CAD build for the part. Positions are in the model's coordinates, mm. A direction names the side the tool comes from. Coordinates: 2 decimals unless noted, no trailing zeros. Write each loop counter-clockwise with the first axis right and the second up, starting at its lowest first coordinate (ties: lowest second). Pieces come first, ordered by that corner, then holes. Notation, with made-up numbers: M -7,-18.5 L 8,-18.5 A16 cw 8,6.5 Z; hole C 3.5,16 d7. An arc over 180 degrees is marked long. Answer as CSV lines item,"result". Start each with the question number.
```python
from build123d import *

# Parameters (mm, degrees)
SKETCH1_R           = 3.5
SKETCH1_R_2         = 1.5
SKETCH1_R_3         = 1.1
EXTRUDE_1_DEPTH     = 3
CUT_EXTRUDE_1_DEPTH = 1.5


with BuildPart() as part:
    # Sketch1 → Бобышка-Вытянуть1 (new body)
    with BuildSketch(Plane.XY):
        with BuildLine():
            Line((-24.498196466, 18.686253871), (-28.812938034, 21.763271713))
            ThreePointArc((-28.812938034, 21.763271713), (-34.033313652, 22.967935089), (-38.576502294, 20.128397731))
            Line((-38.576502294, 20.128397731), (-42.0602267, 15.24335277))
            ThreePointArc((-42.0602267, 15.24335277), (-43.264890076, 10.022977152), (-40.425352718, 5.47978851))
            Line((-40.425352718, 5.47978851), (-36.440527218, 2.638047245))
            ThreePointArc((-36.440527218, 2.638047245), (-34.281914219, 0.144259766), (-33.504872357, -3.061171876))
            Line((-33.504872357, -3.061171876), (-33.504872357, -48.061171876))
            ThreePointArc((-33.504872357, -48.061171876), (-34.969338451, -51.596705782), (-38.504872357, -53.061171876))
            Line((-38.504872357, -53.061171876), (-42.504872357, -53.061171876))
            ThreePointArc((-42.504872357, -53.061171876), (-47.454619825, -55.111424407), (-49.504872357, -60.061171876))
            Line((-49.504872357, -60.061171876), (-49.500334917, -60.235639257))
            Line((-49.500334917, -60.235639257), (-49.500334917, -66.108369799))
            Line((-49.500334917, -66.108369799), (-49.504872357, -66.28283718))
            ThreePointArc((-49.504872357, -66.28283718), (-47.454619825, -71.232584649), (-42.504872357, -73.28283718))
            Line((-42.504872357, -73.28283718), (-38.504872357, -73.28283718))
            ThreePointArc((-38.504872357, -73.28283718), (-34.969338451, -74.747303275), (-33.504872357, -78.28283718))
            Line((-33.504872357, -78.28283718), (-33.504872357, -123.28283718))
            ThreePointArc((-33.504872357, -123.28283718), (-34.281914219, -126.488268823), (-36.440527218, -128.982056301))
            Line((-36.440527218, -128.982056301), (-40.425352718, -131.823797566))
            ThreePointArc((-40.425352718, -131.823797566), (-43.264890076, -136.366986209), (-42.0602267, -141.587361827))
            Line((-42.0602267, -141.587361827), (-38.576502294, -146.472406787))
            ThreePointArc((-38.576502294, -146.472406787), (-34.033313652, -149.311944145), (-28.812938034, -148.107280769))
            Line((-28.812938034, -148.107280769), (-24.498196466, -145.030262927))
            ThreePointArc((-24.498196466, -145.030262927), (-21.740151192, -143.647892601), (-18.691989124, -143.172004528))
            Line((-18.691989124, -143.172004528), (46.687073776, -143.172004528))
            ThreePointArc((46.687073776, -143.172004528), (49.735235844, -143.647892601), (52.493281118, -145.030262927))
            Line((52.493281118, -145.030262927), (56.808022686, -148.107280769))
            ThreePointArc((56.808022686, -148.107280769), (62.028398304, -149.311944145), (66.571586947, -146.472406787))
            Line((66.571586947, -146.472406787), (70.055311352, -141.587361827))
            ThreePointArc((70.055311352, -141.587361827), (71.259974728, -136.366986209), (68.42043737, -131.823797566))
            Line((68.42043737, -131.823797566), (64.43561187, -128.982056301))
            ThreePointArc((64.43561187, -128.982056301), (62.276998871, -126.488268823), (61.499957009, -123.28283718))
            Line((61.499957009, -123.28283718), (61.499957009, -78.28283718))
            ThreePointArc((61.499957009, -78.28283718), (62.964423103, -74.747303275), (66.499957009, -73.28283718))
            Line((66.499957009, -73.28283718), (70.499957009, -73.28283718))
            ThreePointArc((70.499957009, -73.28283718), (75.449704478, -71.232584649), (77.499957009, -66.28283718))
            Line((77.499957009, -66.28283718), (77.495419569, -66.108369799))
            Line((77.495419569, -66.108369799), (77.495419569, -60.235639257))
            Line((77.495419569, -60.235639257), (77.499957009, -60.061171876))
            ThreePointArc((77.499957009, -60.061171876), (75.449704478, -55.111424407), (70.499957009, -53.061171876))
            Line((70.499957009, -53.061171876), (66.499957009, -53.061171876))
            ThreePointArc((66.499957009, -53.061171876), (62.964423103, -51.596705782), (61.499957009, -48.061171876))
            Line((61.499957009, -48.061171876), (61.499957009, -3.061171876))
            ThreePointArc((61.499957009, -3.061171876), (62.276998871, 0.144259766), (64.43561187, 2.638047245))
            Line((64.43561187, 2.638047245), (68.42043737, 5.47978851))
            ThreePointArc((68.42043737, 5.47978851), (71.259974728, 10.022977152), (70.055311352, 15.24335277))
            Line((70.055311352, 15.24335277), (66.571586947, 20.128397731))
            ThreePointArc((66.571586947, 20.128397731), (62.028398304, 22.967935089), (56.808022686, 21.763271713))
            Line((56.808022686, 21.763271713), (52.493281118, 18.686253871))
            ThreePointArc((52.493281118, 18.686253871), (49.735235844, 17.303883544), (46.687073776, 16.827995472))
            Line((46.687073776, 16.827995472), (1.690542794, 16.827995472))
            ThreePointArc((1.690542794, 16.827995472), (1.120947956, 16.649921089), (0.754213617, 16.179118913))
            Line((0.754213617, 16.179118913), (-0.502457674, 12.827995472))
            Line((-0.502457674, 12.827995472), (0.997542326, 12.827995472))
            Line((0.997542326, 12.827995472), (0.997542326, 7.827995472))
            ThreePointArc((0.997542326, 7.827995472), (0.704649107, 7.120888691), (-0.002457674, 6.827995472))
            Line((-0.002457674, 6.827995472), (-1.002457674, 6.827995472))
            ThreePointArc((-1.002457674, 6.827995472), (-1.709564455, 7.120888691), (-2.002457674, 7.827995472))
            Line((-2.002457674, 7.827995472), (-2.002457674, 15.827995472))
            ThreePointArc((-2.002457674, 15.827995472), (-2.295350893, 16.535102253), (-3.002457674, 16.827995472))
            Line((-3.002457674, 16.827995472), (-18.691989124, 16.827995472))
            ThreePointArc((-18.691989124, 16.827995472), (-21.740151192, 17.303883544), (-24.498196466, 18.686253871))
        make_face()
        with Locations((68.745419569, -63.172004528)):
            Circle(SKETCH1_R, mode=Mode.SUBTRACT)
        with Locations((-40.750334917, -63.172004528)):
            Circle(SKETCH1_R, mode=Mode.SUBTRACT)
        with Locations((33.997542326, 10.633411798)):
            Circle(SKETCH1_R_2, mode=Mode.SUBTRACT)
        with Locations((-6.002457674, 10.633411798)):
            Circle(SKETCH1_R_2, mode=Mode.SUBTRACT)
        with Locations((-33.194340596, 12.605443826)):
            Circle(SKETCH1_R, mode=Mode.SUBTRACT)
        with Locations(Location((61.189425248, 12.605443826, 0), (0, 0, 180))):
            Circle(SKETCH1_R, mode=Mode.SUBTRACT)
        with Locations(Location((-6.002457674, -136.977420854, 0), (0, 0, 180))):
            Circle(SKETCH1_R_2, mode=Mode.SUBTRACT)
        with Locations(Location((33.997542326, -136.977420854, 0), (0, 0, 180))):
            Circle(SKETCH1_R_2, mode=Mode.SUBTRACT)
        with Locations((-27.314872357, -100.78283718)):
            Circle(SKETCH1_R_2, mode=Mode.SUBTRACT)
        with Locations((55.309957009, -100.78283718)):
            Circle(SKETCH1_R_2, mode=Mode.SUBTRACT)
        with Locations((-27.314872357, -25.561171876)):
            Circle(SKETCH1_R_2, mode=Mode.SUBTRACT)
        with Locations((55.309957009, -25.561171876)):
            Circle(SKETCH1_R_2, mode=Mode.SUBTRACT)
        with Locations((-12.002457674, -127.18381063)):
            Circle(SKETCH1_R_2, mode=Mode.SUBTRACT)
        with Locations((39.997542326, -127.18381063)):
            Circle(SKETCH1_R_2, mode=Mode.SUBTRACT)
        with Locations((61.189425248, -138.949452883)):
            Circle(SKETCH1_R, mode=Mode.SUBTRACT)
        with Locations(Location((-33.194340596, -138.949452883, 0), (0, 0, 180))):
            Circle(SKETCH1_R, mode=Mode.SUBTRACT)
        with Locations((38.497542326, -76.172004528)):
            Circle(SKETCH1_R_2, mode=Mode.SUBTRACT)
        with Locations((-10.502457674, -76.172004528)):
            Circle(SKETCH1_R_2, mode=Mode.SUBTRACT)
        with Locations((39.997542326, -7.18381063)):
            Circle(SKETCH1_R_2, mode=Mode.SUBTRACT)
        with Locations((-12.002457674, -7.18381063)):
            Circle(SKETCH1_R_2, mode=Mode.SUBTRACT)
        with Locations((3.997542326, -102.172004528)):
            Circle(SKETCH1_R_3, mode=Mode.SUBTRACT)
        with Locations((23.997542326, -102.172004528)):
            Circle(SKETCH1_R_3, mode=Mode.SUBTRACT)
        with Locations((38.497542326, -18.172004528)):
            Circle(SKETCH1_R_2, mode=Mode.SUBTRACT)
        with Locations((-10.502457674, -18.172004528)):
            Circle(SKETCH1_R_2, mode=Mode.SUBTRACT)
        with BuildLine():
            Line((22.997542326, -10.561171876), (26.997542326, -10.561171876))
            ThreePointArc((26.997542326, -10.561171876), (28.411755888, -9.975385438), (28.997542326, -8.561171876))
            Line((28.997542326, -8.561171876), (28.997542326, -0.561171876))
            ThreePointArc((28.997542326, -0.561171876), (27.533076232, 2.97436203), (23.997542326, 4.438828124))
            Line((23.997542326, 4.438828124), (3.997542326, 4.438828124))
            ThreePointArc((3.997542326, 4.438828124), (0.46200842, 2.97436203), (-1.002457674, -0.561171876))
            Line((-1.002457674, -0.561171876), (-1.002457674, -8.561171876))
            ThreePointArc((-1.002457674, -8.561171876), (-0.416671236, -9.975385438), (0.997542326, -10.561171876))
            Line((0.997542326, -10.561171876), (4.997542326, -10.561171876))
            ThreePointArc((4.997542326, -10.561171876), (6.411755888, -11.146958313), (6.997542326, -12.561171876))
            Line((6.997542326, -12.561171876), (6.997542326, -13.561171876))
            ThreePointArc((6.997542326, -13.561171876), (7.583328764, -14.975385438), (8.997542326, -15.561171876))
            Line((8.997542326, -15.561171876), (18.997542326, -15.561171876))
            ThreePointArc((18.997542326, -15.561171876), (20.411755888, -14.975385438), (20.997542326, -13.561171876))
            Line((20.997542326, -13.561171876), (20.997542326, -12.561171876))
            ThreePointArc((20.997542326, -12.561171876), (21.583328764, -11.146958313), (22.997542326, -10.561171876))
        make_face(mode=Mode.SUBTRACT)
    extrude(amount=-EXTRUDE_1_DEPTH)

    # Эскиз1 → Вырез-Вытянуть1 (cut)
    with BuildSketch(Plane(origin=(0, 0, -3), x_dir=(-1, 0, 0), z_dir=(0, 0, -1))):
        Polygon((12.002457674, -4.08381063), (9.317778922, -5.63381063), (9.317778922, -8.73381063), (12.002457674, -10.28381063), (14.687136426, -8.73381063), (14.687136426, -5.63381063), align=None)
        Polygon((-39.997542326, -4.08381063), (-42.682221078, -5.63381063), (-42.682221078, -8.73381063), (-39.997542326, -10.28381063), (-37.312863574, -8.73381063), (-37.312863574, -5.63381063), align=None)
        Polygon((-39.997542326, -130.28381063), (-37.312863574, -128.73381063), (-37.312863574, -125.63381063), (-39.997542326, -124.08381063), (-42.682221078, -125.63381063), (-42.682221078, -128.73381063), align=None)
        Polygon((12.002457674, -130.28381063), (14.687136426, -128.73381063), (14.687136426, -125.63381063), (12.002457674, -124.08381063), (9.317778922, -125.63381063), (9.317778922, -128.73381063), align=None)
    extrude(amount=-CUT_EXTRUDE_1_DEPTH, mode=Mode.SUBTRACT)


solid = part.part
```
1) Band-saw the part on C-C, the plane z = -2.3. State how many separate pieces and enclosed holes the cut face has, plus the area to 3 significant figures.
2) Two-plate mould, pull along Y, no slides. Class faces 4 (the cylindrical face through (-35.008, -74.709, -1.479)), 5 (the flat face through (-40.294, 17.72, -1.479)), 6 (the flat face through (-40.34, -144, -1.48)), 7 (the cylindrical face through (57.851, 11.554, -1.479)): pulls with the +Y half, pulls with the -Y half, needs draft (parallel to the pull), parting line crosses it, or undercut.
3) Pin check, flat tips, straight feed: P1, Ø0.9, axis at y = 10.5, z = -1.5, coming from the +X side; P2, Ø1.5, axis at x = 3.5, z = -1.5, coming from the +Y side; P3, Ø1.5, axis at y = -8, z = -0.5, coming from the -X side. Stop position of each tip, or through.
4) Band-saw the part on B-B, the plane y = -86. List the corners of the cut face in (x, z).
5) Tool access for faces 1 (the flat face through (41, -129, -1.5)), 2 (the cylindrical face through (-34.931, -51.558, -1.479)), 3 (the cylindrical face through (0.5, 3.01, -1.48)): list every direction of +Z, -Z, +X, -X, +Y, -Y with a clear straight run to the whole face (end or side of a thin tool).
6) Band-saw the part on A-A, the plane x = 15. List the corners of the cut face in (y, z), plus the area to 3 significant figures.
7) Probe L1, parallel to Y at x = 25, z = -2.5; L2, parallel to Y at x = -10, z = -1.35; L3, parallel to X at y = -62, z = -0.15. List the from-to ranges inside material, lowest first. Write a range as [from, to].
Result sheet:
1,separate pieces,"1"
1,enclosed holes,"25"
1,area,"15,700 mm²"
2,face 4,"undercut"
2,face 5,"pulls with the +Y half"
2,face 6,"pulls with the -Y half"
2,face 7,"undercut"
3,P1,"stops at x = 71.35"
3,P2,"stops at y = 16.83"
3,P3,"stops at x = -33.5"
4,outline,"M -33.5,-3 L 61.5,-3 L 61.5,0 L -33.5,0 Z"
5,face 1,"-Z"
5,face 2,"+Z, -Z, -X"
5,face 3,"+Z, -Z"
6,outline,"M -143.17,-3 L -15.56,-3 L -15.56,0 L -143.17,0 Z; M 4.44,-3 L 16.83,-3 L 16.83,0 L 4.44,0 Z"
6,area,"420 mm²"
7,L1,"y = [-143.17, -102.62], [-101.72, -10.56], [4.34, 16.83]"
7,L2,"y = [-143.17, -77.59], [-74.76, -19.59], [-16.76, 16.83]"
7,L3,"x = [-49.5, -44.05], [-37.45, 65.45], [72.04, 77.5]"
